from build123d import *

# Parameters (mm, degrees)
BRIDA_BASE1_DEPTH           = 48
CROQUIS5_R                  = 2.5
CORTAR_EXTRUIR1_DEPTH       = 10
CORTAR_EXTRUIR2_START       = 28
CORTAR_EXTRUIR2_DEPTH       = 20
CORTAR_EXTRUIR2_2_DEPTH     = 10
CORTAR_EXTRUIR2_START_2     = -38.506869712
CORTAR_EXTRUIR2_3_OUTLINE_R = 1.5
CORTAR_EXTRUIR2_3_DEPTH     = 14.5
CROQUIS7_W                  = 12.5
CROQUIS7_H                  = 4
CORTAR_EXTRUIR4_DEPTH       = 10


with BuildPart() as part:
    # Brida base1: sheet metal written as solids
    # Croquis1 → Brida base1 (new body)
    with BuildSketch(Plane.XY):
        with BuildLine():
            Line((-38.506869712, -5.805989848), (-38.506869712, -12.555989848))
            ThreePointArc((-38.506869712, -12.555989848), (-38.213976494, -13.263096629), (-37.506869712, -13.555989848))
            Line((-37.506869712, -13.555989848), (-25.006869712, -13.555989848))
            ThreePointArc((-25.006869712, -13.555989848), (-24.299762931, -13.263096629), (-24.006869712, -12.555989848))
            Line((-24.006869712, -12.555989848), (-24.006869712, -5.805989848))
            Line((-24.006869712, -5.805989848), (-24.506869712, -5.805989848))
            Line((-24.506869712, -5.805989848), (-24.506869712, -12.555989848))
            ThreePointArc((-24.506869712, -12.555989848), (-24.653316322, -12.909543238), (-25.006869712, -13.055989848))
            Line((-25.006869712, -13.055989848), (-37.506869712, -13.055989848))
            ThreePointArc((-37.506869712, -13.055989848), (-37.860423103, -12.909543238), (-38.006869712, -12.555989848))
            Line((-38.006869712, -12.555989848), (-38.006869712, -5.805989848))
            Line((-38.006869712, -5.805989848), (-38.506869712, -5.805989848))
        make_face()
    extrude(amount=BRIDA_BASE1_DEPTH)

    # Croquis5 → Cortar-Extruir1 (cut)
    with BuildSketch(Plane(origin=(0, -13.055989848, 0), x_dir=(1, 0, 0), z_dir=(0, 1, 0))):
        with Locations(Location((-31.256869712, -38, 0), (0, 0, 180))):
            Circle(CROQUIS5_R)
    extrude(amount=-CORTAR_EXTRUIR1_DEPTH, mode=Mode.SUBTRACT)

    # Cortar-Extruir2: read off the stored shape, not the designer's step
    # Cortar-Extruir2 outline → Cortar-Extruir2 (cut)
    with BuildSketch(Plane.XY.offset(CORTAR_EXTRUIR2_START)):
        with BuildLine():
            Line((-37.506869712, -13.555989848), (-37.506869712, -13.055989848))
            ThreePointArc((-37.506869712, -13.055989848), (-37.860423103, -12.909543239), (-38.006869712, -12.555989848))
            Line((-38.006869712, -12.555989848), (-38.006869712, -5.805989848))
            Line((-38.006869712, -5.805989848), (-38.506869712, -5.805989848))
            Line((-38.506869712, -5.805989848), (-38.506869712, -12.555989848))
            ThreePointArc((-38.506869712, -12.555989848), (-38.213976493, -13.26309663), (-37.506869712, -13.555989848))
        make_face()
        with BuildLine():
            ThreePointArc((-24.506869712, -12.555989848), (-24.653316322, -12.909543238), (-25.006869712, -13.055989848))
            Line((-25.006869712, -13.055989848), (-25.006869712, -13.555989848))
            ThreePointArc((-25.006869712, -13.555989848), (-24.299762931, -13.263096629), (-24.006869712, -12.555989848))
            Line((-24.006869712, -12.555989848), (-24.006869712, -5.805989848))
            Line((-24.006869712, -5.805989848), (-24.506869712, -5.805989848))
            Line((-24.506869712, -5.805989848), (-24.506869712, -12.555989848))
        make_face()
    extrude(amount=CORTAR_EXTRUIR2_DEPTH, mode=Mode.SUBTRACT)

    # Cortar-Extruir2 2 outline → Cortar-Extruir2 2 (cut)
    with BuildSketch(Plane.XY):
        with BuildLine():
            Line((-37.506869712, -13.555989848), (-37.506869712, -13.055989848))
            ThreePointArc((-37.506869712, -13.055989848), (-37.860423103, -12.909543239), (-38.006869712, -12.555989848))
            Line((-38.006869712, -12.555989848), (-38.006869712, -5.805989848))
            Line((-38.006869712, -5.805989848), (-38.506869712, -5.805989848))
            Line((-38.506869712, -5.805989848), (-38.506869712, -12.555989848))
            ThreePointArc((-38.506869712, -12.555989848), (-38.213976493, -13.26309663), (-37.506869712, -13.555989848))
        make_face()
        with BuildLine():
            ThreePointArc((-24.506869712, -12.555989848), (-24.653316322, -12.909543238), (-25.006869712, -13.055989848))
            Line((-25.006869712, -13.055989848), (-25.006869712, -13.555989848))
            ThreePointArc((-25.006869712, -13.555989848), (-24.299762931, -13.263096629), (-24.006869712, -12.555989848))
            Line((-24.006869712, -12.555989848), (-24.006869712, -5.805989848))
            Line((-24.006869712, -5.805989848), (-24.506869712, -5.805989848))
            Line((-24.506869712, -5.805989848), (-24.506869712, -12.555989848))
        make_face()
    extrude(amount=CORTAR_EXTRUIR2_2_DEPTH, mode=Mode.SUBTRACT)

    # Cortar-Extruir2 3 outline → Cortar-Extruir2 3 (cut)
    with BuildSketch(Plane.YZ.offset(CORTAR_EXTRUIR2_START_2)):
        with Locations((-9.805989848, 23)):
            Circle(CORTAR_EXTRUIR2_3_OUTLINE_R)
        with Locations((-9.805989848, 15)):
            Circle(CORTAR_EXTRUIR2_3_OUTLINE_R)
    extrude(amount=CORTAR_EXTRUIR2_3_DEPTH, mode=Mode.SUBTRACT)

    # Croquis7 → Cortar-Extruir4 (cut)
    with BuildSketch(Plane(origin=(0, -13.055989848, 0), x_dir=(1, 0, 0), z_dir=(0, 1, 0))):
        with Locations((-31.256869712, -2)):
            Rectangle(CROQUIS7_W, CROQUIS7_H)
    extrude(amount=-CORTAR_EXTRUIR4_DEPTH, mode=Mode.SUBTRACT)


solid = part.part
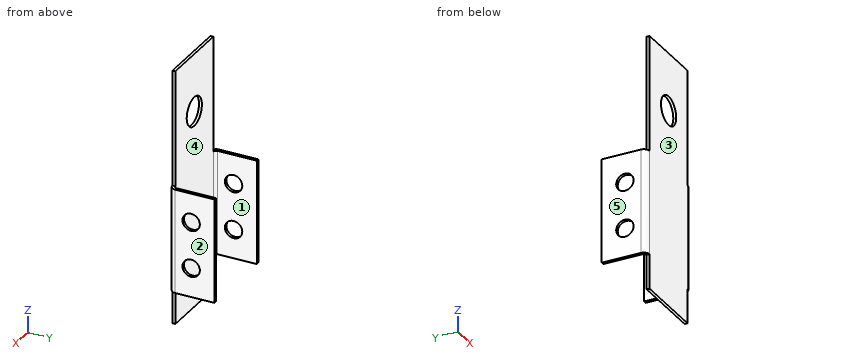
Geometry check sheet. Reference: the model listing, model coordinates, mm. Face numbers are marked on the shaded views. A direction names the side the tool comes from. Round coordinates to 2 decimals unless told otherwise and drop trailing zeros. Order: outer loops, then holes, each group sorted by start corner. A loop starts at its lowest first (then second) coordinate and runs counter-clockwise, first axis right, second up. Notation, with made-up numbers: M 6,85.5 L 29,85.5 A9 cw 29,102.5 Z; hole C 19,-37 d10. An arc over 180 degrees is marked long. Answer in a Markdown table with one row per item.
(1) Tool access check on the marked faces 4 and 5. Record the directions out of +Z, -Z, +X, -X, +Y, -Y that give a thin tool (end or side, any length) a straight path to the whole face; none if there is none.
Responses:
| item | result |
|---|---|
| face 4 | +Z, -Z, +Y |
| face 5 | +Z, -Z, -X, +Y, -Y |
(2) Draft check along X on the marked faces 1, 2 and 3. Enter one of: released by +X, released by -X, zero draft, split by the parting line, or undercut.
Responses:
| item | result |
|---|---|
| face 1 | undercut |
| face 2 | released by +X |
| face 3 | zero draft |
(3) Sectioned sample at A-A, the plane z = 15. Record the cut outline in (x, y).
Responses:
| item | result |
|---|---|
| outline | M -38.51,-12.56 A1 ccw -37.51,-13.56 L -25.01,-13.56 A1 ccw -24.01,-12.56 L -24.01,-11.31 L -24.51,-11.31 L -24.51,-12.56 A0.5 cw -25.01,-13.06 L -37.51,-13.06 A0.5 cw -38.01,-12.56 L -38.01,-11.31 L -38.51,-11.31 Z; M -38.51,-8.31 L -38.01,-8.31 L -38.01,-5.81 L -38.51,-5.81 Z; M -24.51,-8.31 L -24.01,-8.31 L -24.01,-5.81 L -24.51,-5.81 Z |
(4) Sectioned sample at D-D, the plane y = -9.75. Record the cut outline in (x, z).
Responses:
| item | result |
|---|---|
| outline | M -38.51,10 L -38.01,10 L -38.01,13.5 L -38.51,13.5 Z; M -38.51,16.5 L -38.01,16.5 L -38.01,21.5 L -38.51,21.5 Z; M -38.51,24.5 L -38.01,24.5 L -38.01,28 L -38.51,28 Z; M -24.51,10 L -24.01,10 L -24.01,13.5 L -24.51,13.5 Z; M -24.51,16.5 L -24.01,16.5 L -24.01,21.5 L -24.51,21.5 Z; M -24.51,24.5 L -24.01,24.5 L -24.01,28 L -24.51,28 Z |
(5) Go/stop test with flat-tipped pins: P1, Ø0.6, axis at y = -13.5, z = 8, coming from the +X side; P2, Ø6.5, axis at x = -31.26, z = 38, coming from the +Y side; P3, Ø1.1, axis at x = -24.5, y = -9.5, coming from the -Z side. Record where each tip stops, or that it passes through.
Responses:
| item | result |
|---|---|
| P1 | stops at x = -25.01 |
| P2 | stops at y = -13.06 |
| P3 | stops at z = 10 |
(6) Sectioned sample at B-B, the plane y = -6.25. Record the cut outline in (x, z).
Responses:
| item | result |
|---|---|
| outline | M -38.51,10 L -38.01,10 L -38.01,28 L -38.51,28 Z; M -24.51,10 L -24.01,10 L -24.01,28 L -24.51,28 Z |
(7) Scan lines: probe 1 along X at (y, z) = (-9.25, 19.5); probe 2 along Y at (x, z) = (-27.75, 26); probe 3 along Y at (x, z) = (-24.3, 23). Record each from-to range of solid material in increasing order. Write a range as from..to.
Responses:
| item | result |
|---|---|
| probe 1 | x = -38.51..-38.01, -24.51..-24.01 |
| probe 2 | y = -13.56..-13.06 |
| probe 3 | y = -13.26..-11.31, -8.31..-5.81 |
(8) Sectioned sample at C-C, the plane z = 38. Record the cut outline in (x, y), and give its area (3 significant figures).
Responses:
| item | result |
|---|---|
| outline | M -37.51,-13.56 L -33.76,-13.56 L -33.76,-13.06 L -37.51,-13.06 Z; M -28.76,-13.56 L -25.01,-13.56 L -25.01,-13.06 L -28.76,-13.06 Z |
| area | 3.75 mm² |
